The drawing under review shows one solid part. Ordinate dimensions are in mm from its lowest x, y, z. A direction names the side the tool comes from. Coordinates: 2 decimals unless noted, no trailing zeros. Order: outer loops, then holes, each group sorted by start corner. A loop starts at its lowest first (then second) coordinate and runs counter-clockwise, first axis right, second up. Notation, with made-up numbers: (67.25, 87) -> (118.25, 87) arc R9 ccw to (118.25, 92) -> close; hole circle Ø5 at (49, 46). An arc over 180 degrees is marked (long way). Put each result on its own line as item: value.
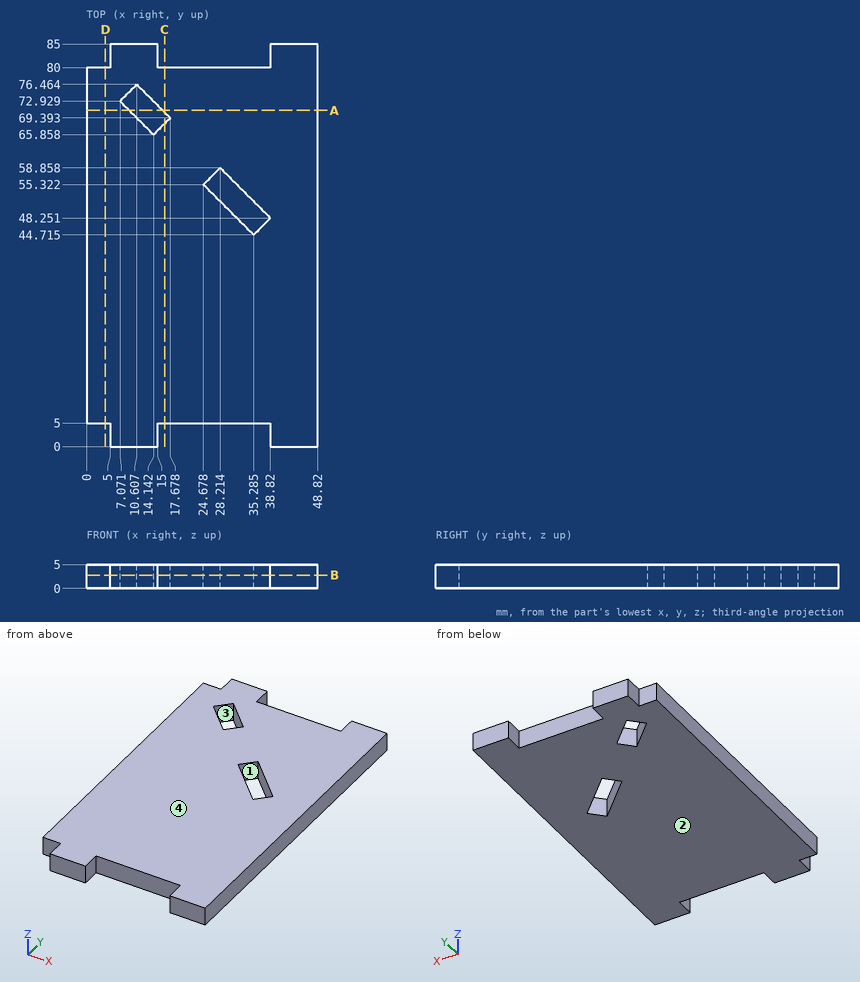
Item 1: Consider section B-B on z = 2.8. Count the separate pieces of the cut face and the enclosed holes in it, and give its area (3 significant figures).
Answers below:
separate pieces: 1
enclosed holes: 2
area: 3,740 mm^2
Item 2: Consider section C-C on x = 16.5. Write out the cut boundary in (y, z) (1 decimal).
Answers below:
outline: (5, 0) -> (68.2, 0) -> (68.2, 5) -> (5, 5) -> close; (70.6, 0) -> (80, 0) -> (80, 5) -> (70.6, 5) -> close
Item 3: Consider section A-A on y = 71. Write out the cut boundary in (x, z).
Answers below:
outline: (0, 0) -> (9, 0) -> (9, 5) -> (0, 5) -> close; (16.07, 0) -> (48.82, 0) -> (48.82, 5) -> (16.07, 5) -> close
Item 4: For line 1 (Y direction, x = 18.5, z = 3.3); line 2 (X direction, y = 53, z = 2.65); line 3 (Y direction, x = 34, z = 3.35), list the stretches that pass through material, from the lowest coordinate up. Write a range as from..to.
Answers below:
line 1: 5..80
line 2: 0..27, 34.07..48.82
line 3: 5..46, 53.07..80
Item 5: For pin 1 Ø2.5 at (x, z) = (3.5, 2.5) entering from -Y; pin 2 Ø2.5 at (y, z) = (83.5, 1.5) entering from -X; pin 3 Ø2.5 at (x, z) = (26, 2) entering from +Y, all flat-tipped, find the tip position at first contact; note any pin that passes through.
Answers below:
pin 1: y = 5
pin 2: x = 5
pin 3: y = 80
Item 6: For the marked faces 3 and 4, list the 3-axis set-ups (+Z, -Z, +X, -X, +Y, -Y) from which the entire face can be reached by the end or side of a thin tool; tool diameter is ignored.
Answers below:
face 3: +Z, -Z
face 4: +Z, +X, -X, +Y, -Y
Item 7: Consider section D-D on x = 4. Write out the cut boundary in (y, z).
Answers below:
outline: (5, 0) -> (80, 0) -> (80, 5) -> (5, 5) -> close
Item 8: Mouldability with a two-part tool opening along Y and no side actions: class the marked faces 1 and 2 as +Y half, -Y half, draft (parallel to the pull), parting line (faces both ways), or undercut.
Answers below:
face 1: undercut
face 2: draft
